Could you check a few things on this drawing? It's one solid part, dimensions in mm from its lowest x, y, z. A direction names the side the tool comes from. Coordinates: 2 decimals unless noted, no trailing zeros. Write each loop counter-clockwise with the first axis right and the second up, starting at its lowest first coordinate (ties: lowest second). Pieces come first, ordered by that corner, then holes. Notation, with made-up numbers: (45.5, -5.5) - (68.5, -5.5) arc R18 ccw to (68.5, -0.5) - close; hole circle Ø4 at (55, 79.5). An arc over 180 degrees is marked (long way). Use one line per item in the form item = value. Start each with the question number.
(1) For pin 1 Ø3 at (x, z) = (22.8, 14.6) entering from +Y; pin 2 Ø3.5 at (x, z) = (20, 13) entering from +Y, each with a flat end and sliding along its axis, tell me the tip position at first contact or that it passes through.
(2) If we section it at D-D on x = 19: Please give me the cut outline in (y, z), then the cut area to 3 significant figures.
(3) If we section it at B-B on x = 13: Please give me the cut outline in (y, z).
(4) On a 3-axis mill with a long thin cutter (end or side, diameter ignored), from which of +Z, -Z, +X, -X, +Y, -Y can I reach the whole of each face in a straight line? I mean the marked faces 1 and 2. Say none if no direction works.
(5) If I drill on probe 1 along Y at (x, z) = (31.59, 18.25); probe 2 along X at (y, z) = (15, 19) (1 decimal); probe 3 along X at (y, z) = (17, 5.75), over which ranges is the centre line in solid material (lowest first)? Write a range as from..to.
(6) If we section it at A-A on z = 20.75: Please give me the cut outline in (x, y), then the cut area to 3 significant figures.
(7) If we section it at C-C on y = 6: Please give me the cut outline in (x, z), then the cut area to 3 significant figures.
(8) Thinking about a two-plate mould opening in Y: for the marked faces 3, 4 and 5, which applies, pulls with the +Y half, pulls with the -Y half, needs draft (parallel to the pull), parting line crosses it, or undercut?
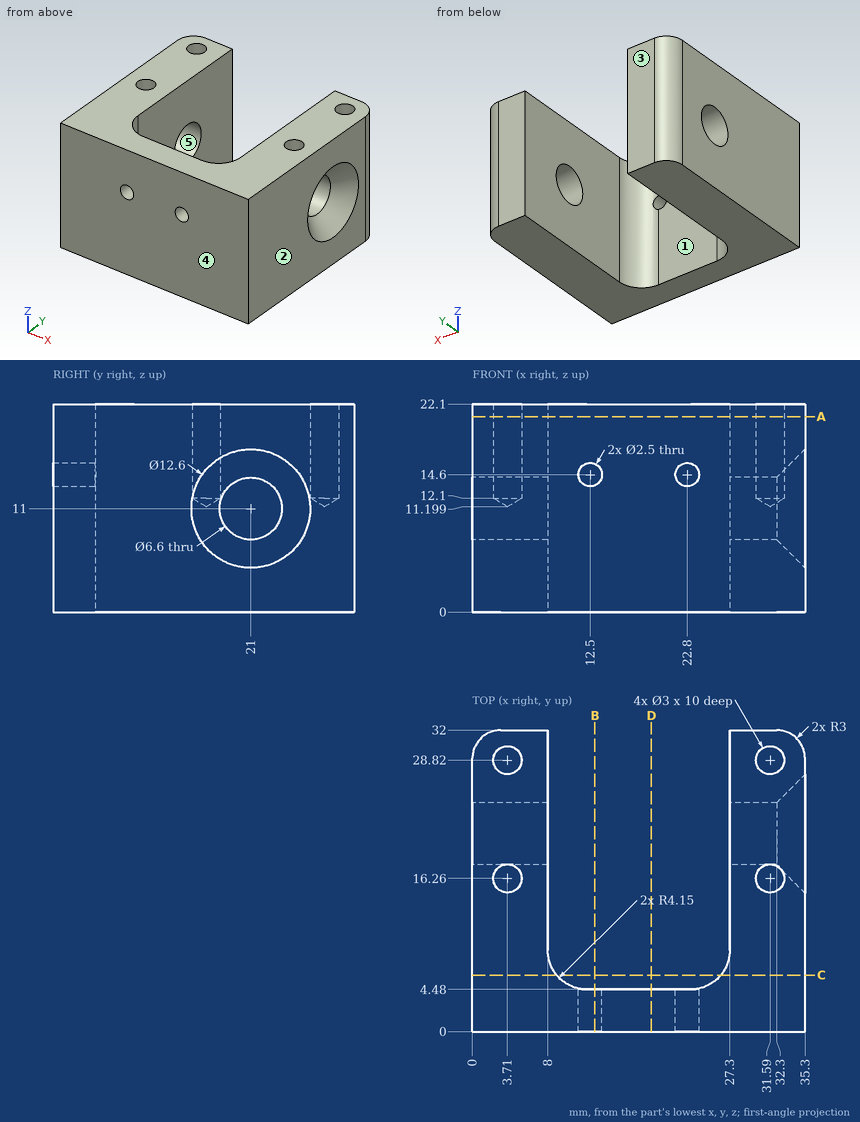
Reported:
q1.pin_1 = 4.64
q1.pin_2 = 4.48
q2.outline = (0, 0) - (4.48, 0) - (4.48, 22.1) - (0, 22.1) - close
q2.area = 99.0 mm2
q3.outline = (0, 0) - (4.48, 0) - (4.48, 13.45) - (0, 13.45) - close; (0, 15.75) - (4.48, 15.75) - (4.48, 22.1) - (0, 22.1) - close
q4.face_1 = +Z, -Z, +Y
q4.face_2 = +Z, -Z, +X, +Y, -Y
q5.probe_1 = 0..14.76, 17.76..27.32, 30.32..32
q5.probe_2 = 0..2.9, 4.5..8, 27.3..30.8, 32.4..35.3
q5.probe_3 = 0..8, 27.3..35.3
q6.outline = (0, 0) - (35.3, 0) - (35.3, 29) arc R3 ccw to (32.3, 32) - (27.3, 32) - (27.3, 8.63) arc R4.15 cw to (23.15, 4.48) - (12.15, 4.48) arc R4.15 cw to (8, 8.63) - (8, 32) - (3, 32) arc R3 ccw to (0, 29) - close; hole circle Ø3 at (3.71, 16.26); hole circle Ø3 at (3.71, 28.82); hole circle Ø3 at (31.59, 16.26); hole circle Ø3 at (31.59, 28.82)
q6.area = 574 mm2
q7.outline = (0, 0) - (8.94, 0) - (8.94, 22.1) - (0, 22.1) - close; (26.36, 0) - (35.3, 0) - (35.3, 22.1) - (26.36, 22.1) - close
q7.area = 395 mm2
q8.face_3 = pulls with the +Y half
q8.face_4 = pulls with the -Y half
q8.face_5 = undercut
